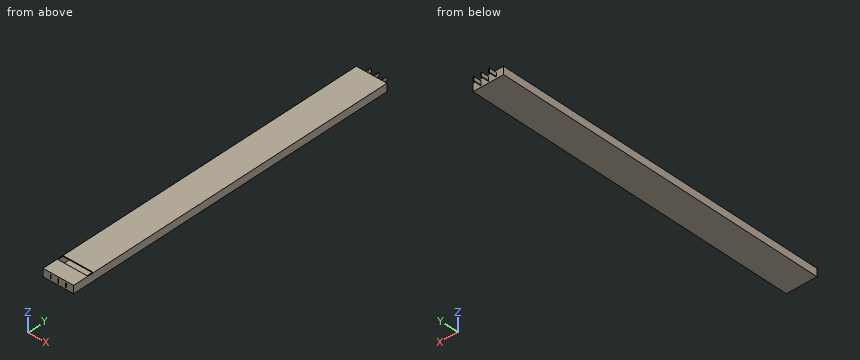
from build123d import *

# Parameters (mm, degrees)
SKETCH2_W           = 40
SKETCH2_H           = 10
BOSS_EXTRUDE2_DEPTH = 440
SKETCH3_W           = 38
SKETCH3_H           = 8
CUT_EXTRUDE1_DEPTH  = 438
BOSS_EXTRUDE4_DEPTH = 10
LPATTERN2_COUNT     = 3
LPATTERN2_PITCH     = 10
SKETCH5_W           = 38
SKETCH5_H           = 8
BOSS_EXTRUDE5_DEPTH = 12
CUT_EXTRUDE2_DEPTH  = 11
LPATTERN3_COUNT     = 3
LPATTERN3_PITCH     = 10
SKETCH7_W           = 38
SKETCH7_H           = 8
CUT_EXTRUDE3_DEPTH  = 5


with BuildPart() as part:
    # Sketch2 → Boss-Extrude2 (new body)
    with BuildSketch(Plane(origin=(0, 0, 0), x_dir=(1, 0, 0), z_dir=(0, 1, 0))):
        Rectangle(SKETCH2_W, SKETCH2_H)
    extrude(amount=BOSS_EXTRUDE2_DEPTH)

    # Sketch3 → Cut-Extrude1 (cut)
    with BuildSketch(Plane(origin=(0, 0, 0), x_dir=(1, 0, 0), z_dir=(0, 1, 0))):
        Rectangle(SKETCH3_W, SKETCH3_H)
    extrude(amount=CUT_EXTRUDE1_DEPTH, mode=Mode.SUBTRACT)

    # Sketch4 → Boss-Extrude4 (add)
    with BuildSketch(Plane(origin=(0, 440, 0), x_dir=(1, 0, 0), z_dir=(0, 1, 0))):
        with BuildLine():
            Line((-10.5, -2.25), (-10.5, 2.25))
            ThreePointArc((-10.5, 2.25), (-10, 2.75), (-9.5, 2.25))
            Line((-9.5, 2.25), (-9.5, -2.25))
            ThreePointArc((-9.5, -2.25), (-10, -2.75), (-10.5, -2.25))
        make_face()
    boss_extrude4 = extrude(amount=BOSS_EXTRUDE4_DEPTH)

    # LPattern2: Boss-Extrude4 ×3
    with Locations(*[(i * LPATTERN2_PITCH, 0, 0) for i in range(1, LPATTERN2_COUNT)]):
        add(boss_extrude4)

    # Sketch5 → Boss-Extrude5 (add)
    with BuildSketch(Plane(origin=(0, 0, 0), x_dir=(-1, 0, 0), z_dir=(0, -1, 0))):
        Rectangle(SKETCH5_W, SKETCH5_H)
    extrude(amount=-BOSS_EXTRUDE5_DEPTH)

    # Sketch6 → Cut-Extrude2 (cut)
    with BuildSketch(Plane.XZ):
        with BuildLine():
            Line((10.5, 2.25), (10.5, -2.25))
            ThreePointArc((10.5, -2.25), (10, -2.75), (9.5, -2.25))
            Line((9.5, -2.25), (9.5, 2.25))
            ThreePointArc((9.5, 2.25), (10, 2.75), (10.5, 2.25))
        make_face()
    cut_extrude2 = extrude(amount=-CUT_EXTRUDE2_DEPTH, mode=Mode.SUBTRACT)

    # LPattern3: Cut-Extrude2 ×3
    with Locations(*[(-i * LPATTERN3_PITCH, 0, 0) for i in range(1, LPATTERN3_COUNT)]):
        add(cut_extrude2, mode=Mode.SUBTRACT)

    # Sketch7 → Cut-Extrude3 (cut)
    with BuildSketch(Plane.XY.offset(5)):
        with Locations((0, 24)):
            Rectangle(SKETCH7_W, SKETCH7_H)
    extrude(amount=-CUT_EXTRUDE3_DEPTH, mode=Mode.SUBTRACT)


solid = part.part
Could you check a few things on this model? Use its own coordinates, in mm. Give positions to 0.01 mm unless a question says otherwise; leave off trailing zeros. Order: outer loops, then holes, each group sorted by start corner. A loop starts at its lowest first (then second) coordinate and runs counter-clockwise, first axis right, second up.
Item 1: I'm going to push flat-ended pins straight in: pin 1 (2 mm diameter, centred on y = 447, z = 0, fed in from -X); pin 2 (3.5 mm diameter, centred on y = 446.5, z = -1, fed in from +X); pin 3 (1.1 mm diameter, centred on x = 9, z = 4.5, fed in from +Y). Where does each tip first touch, or does it pass through?
Item 2: If we section it at A-A, the plane y = 383.5: Write out the boundary of the cut face in (x, z), plus the area to 3 significant figures.
Item 3: I need wall thicknesses on line 1 (X direction, y = 194, z = -3); line 2 (Z direction, x = 1, y = 422.5); line 3 (Y direction, x = 14.5, z = 4.5). Which ranges of each line are inside material? Lowest first, please.
Values:
1. pin 1: stops at x = -10.5
1. pin 2: stops at x = 10.5
1. pin 3: stops at y = 440
2. outline: (-20, -5) - (20, -5) - (20, 5) - (-20, 5) - close; hole (-19, -4) - (19, -4) - (19, 4) - (-19, 4) - close
2. area: 96.0 mm2
3. line 1: x = -20 to -19, 19 to 20
3. line 2: z = -5 to -4, 4 to 5
3. line 3: y = 0 to 20, 28 to 440
